Design review of the part built by this model. Coordinates are the model's own, in mm. A direction names the side the tool comes from. Give positions to 0.01 mm unless a question says otherwise; leave off trailing zeros. Write each loop counter-clockwise with the first axis right and the second up, starting at its lowest first coordinate (ties: lowest second). Pieces come first, ordered by that corner, then holes. Notation, with made-up numbers: (13, 15) - (26, 15) arc R26 cw to (26, 53) - close; hole circle Ø11 at (86.5, -36). An arc over 180 degrees is marked (long way). Write each question's results on one line, items separated by ' | '. Start each with the question number.
from build123d import *

# Parameters (mm, degrees)
F1_ANGLE       = 359
F3_DEPTH       = 4
F5_D           = 3.3
F5_DEPTH       = 8
F5_CSINK_D     = 5
F5_CSINK_ANGLE = 90
F5_TIP         = 0.9914200214
F6_R           = 2.15
F7_DEPTH       = 8
F8_R           = 1


with BuildPart() as f1:
    # F0 (on Front) → F1 (revolve)
    with BuildSketch(Plane.XZ):
        Polygon((38.5, 4), (40.5, 2), (40.5, -2), (38.5, -4), (43.5, -4), (43.5, 4), align=None)
    revolve(axis=Axis((0, 0, 13.8600002974), (0, 0, 1)), revolution_arc=F1_ANGLE)

    # F2 (on Top) → F3 (join, symmetric)
    with BuildSketch(Plane.XY):
        Polygon((42.7580401796, 8), (42.6183996602, 0), (43.5, 0), (51.5, 0), (51.5, 8), align=None)
        Polygon((42.5800298362, -0.7432371854), (42.5800298362, -8.8989358438), (51.5, -8.8989358438), (51.5, -0.8989358438), (43.4933747393, -0.75917968), align=None)
    extrude(amount=F3_DEPTH, both=True)

    # F5
    with Locations(Plane.XZ.offset(8.8989358438)):
        with Locations((47.0400149181, 0)):
            CounterSinkHole(F5_D / 2, F5_CSINK_D / 2, depth=F5_DEPTH, counter_sink_angle=F5_CSINK_ANGLE)
            with Locations((0, 0, -(F5_DEPTH + F5_TIP / 2))):  # 118° drill point
                Cone(0, F5_D / 2, F5_TIP, mode=Mode.SUBTRACT)

    # F6 (on face) → F7 (cut, through all)
    with BuildSketch(Plane(origin=(0, 8, 0), x_dir=(-1, 0, 0), z_dir=(0, 1, 0))):
        with Locations((-47.1290200898, 0)):
            Circle(F6_R)
    extrude(amount=-F7_DEPTH, mode=Mode.SUBTRACT)

    # F8
    f8_edges = [f1.edges().sort_by_distance(p)[0] for p in [
        (47.12902, 8, -4),
        (-43.497587, 0.458196, -4),
        (51.5, 4, -4),
        (51.5, -4.898936, -4),
        (47.040015, -8.898936, -4),
        (51.5, 4, 4),
        (47.12902, 8, 4),
        (-43.497587, 0.458196, 4),
        (47.040015, -8.898936, 4),
        (51.5, -4.898936, 4),
        (51.5, -8.898936, 0),
        (51.5, 8, 0),
        (42.75804, 8, 0),
        (42.58003, -8.898936, 0),
    ]]
    fillet(f8_edges, radius=F8_R)


solid = f1.part
Q1. The part is to be moulded in two halves that separate along Z. For faces 5 (the face through (-40.444, 2.129, -0.028)), 6 (the face through (51.5, -4, 0)), 7 (the face through (38.2, 6.5, 4)), say which applies: +Z half, -Z half, draft (parallel to the pull), parting line (faces both ways), or undercut.
Q2. Insertion check: P1, Ø4, axis at x = 47.04, z = 0, coming from the -Y side; P2, Ø1.5, axis at x = 10.5, z = 1.5, coming from the +Y side; P3, Ø1.5, axis at y = -29, z = -2.5, coming from the +X side. Each pin has a flat end and moves straight along its axis. Give the tip position at first contact, or say it passes through.
Q3. Machinability: for faces 1 (the face through (44.8, 8, 0)), 2 (the face through (45, -8.899, -2)), 3 (the face through (48.69, -4.42, 0.07)), 4 (the face through (45, 0, 1)), which of the approach directions +Z, -Z, +X, -X, +Y, -Y give a long, thin tool a straight path to every point of the face, cutting with its end or side? Answer none if there is none.
Q4. For line 1 along X through (y, z) = (-2.75, 0); line 2 along X through (y, z) = (-6.5, 0) (3 decimals); line 3 along X through (y, z) = (1, 2.5), list the stretches that pass through material, from the lowest coordinate up. Write a range as [from, to].
Q5. Add section A-A on x = 0. State the section outline as (y, z) points, plus the area to 3 significant figures.
Result:
1) face 5: undercut | face 6: draft | face 7: +Z half
2) P1: stops at y = -8.4 | P2: stops at y = 42.39 | P3: stops at x = 33.08
3) face 1: +Z, -Z, +X, +Y | face 2: +Z, -Z, +X, -Y | face 3: -Y | face 4: +Z, -Z, +X
4) line 1: x = [-43.41, -40.41], [40.41, 45.39], [48.69, 51.5] | line 2: x = [-43.012, -39.975], [39.975, 45.39], [48.69, 51.5] | line 3: x = [-43.49, -39.99], [39.99, 51.5]
5) outline: (-43.5, -3) arc R1 ccw to (-42.5, -4) - (-38.5, -4) - (-40.5, -2) - (-40.5, 2) - (-38.5, 4) - (-42.5, 4) arc R1 ccw to (-43.5, 3) - close; (38.5, -4) - (42.5, -4) arc R1 ccw to (43.5, -3) - (43.5, 3) arc R1 ccw to (42.5, 4) - (38.5, 4) - (40.5, 2) - (40.5, -2) - close | area: 55.1 mm²
